```python
from build123d import *

# Parameters (mm, degrees)
BOSS_EXTRUDE1_DEPTH = 18
CIRPATTERN1_COUNT   = 3
SKETCH4_R           = 1.75
CUT_EXTRUDE1_DEPTH  = 12
CIRPATTERN2_COUNT   = 3
SKETCH5_R           = 1.75
CUT_EXTRUDE2_DEPTH  = 44.819230938
CIRPATTERN3_COUNT   = 3


with BuildPart() as part:
    # Sketch2 → Revolve1 (revolve)
    with BuildSketch(Plane(origin=(0, 0, 0), x_dir=(0, 0, -1), z_dir=(1, 0, 0)), mode=Mode.PRIVATE) as revolve1_sk:
        Polygon((0, 28.25), (-3, 28.25), (-3, 18.5), (0, 18.5), (4, 18.5), (4, 28.25), align=None)
    revolve(revolve1_sk.sketch.rotate(Axis((0, 0, 0), (0, 0, 1)), 90), axis=Axis((0, 0, 0), (0, 0, 1)))

    # Sketch3 → Boss-Extrude1 (add)
    with BuildSketch(Plane.XY.offset(3)):
        with BuildLine():
            Line((-7.524627897, 16.900590966), (-11.490310167, 25.807659178))
            ThreePointArc((-11.490310167, 25.807659178), (0, 28.25), (11.490310167, 25.807659178))
            Line((11.490310167, 25.807659178), (7.524627897, 16.900590966))
            ThreePointArc((7.524627897, 16.900590966), (0, 18.5), (-7.524627897, 16.900590966))
        make_face()
    boss_extrude1 = extrude(amount=BOSS_EXTRUDE1_DEPTH)

    # CirPattern1: Boss-Extrude1 ×3 about axis
    cirpattern1_axis = Axis((0, 0, 0), (0, 0, 1))
    for i in range(1, CIRPATTERN1_COUNT):
        add(boss_extrude1.rotate(cirpattern1_axis, i * 360 / CIRPATTERN1_COUNT))

    # Sketch4 → Cut-Extrude1 (cut)
    with BuildSketch(Plane.XY.offset(21)):
        with Locations((0, 23.25)):
            Circle(SKETCH4_R)
    cut_extrude1 = extrude(amount=-CUT_EXTRUDE1_DEPTH, mode=Mode.SUBTRACT)

    # CirPattern2: Cut-Extrude1 ×3 about axis
    cirpattern2_axis = Axis((0, 0, 0), (0, 0, 1))
    for i in range(1, CIRPATTERN2_COUNT):
        add(cut_extrude1.rotate(cirpattern2_axis, i * 360 / CIRPATTERN2_COUNT), mode=Mode.SUBTRACT)

    # Sketch5 → Cut-Extrude2 (cut, through all)
    with BuildSketch(Plane.XY.offset(3)):
        with Locations((0, -23.25)):
            Circle(SKETCH5_R)
    cut_extrude2 = extrude(amount=-CUT_EXTRUDE2_DEPTH, mode=Mode.SUBTRACT)

    # CirPattern3: Cut-Extrude2 ×3 about axis
    cirpattern3_axis = Axis((0, 0, 0), (0, 0, 1))
    for i in range(1, CIRPATTERN3_COUNT):
        add(cut_extrude2.rotate(cirpattern3_axis, i * 360 / CIRPATTERN3_COUNT), mode=Mode.SUBTRACT)


solid = part.part
```
Design review of the part built by this model. Coordinates are the model's own, in mm. A direction names the side the tool comes from. Coordinates: 2 decimals unless noted, no trailing zeros. Order: outer loops, then holes, each group sorted by start corner. A loop starts at its lowest first (then second) coordinate and runs counter-clockwise, first axis right, second up.
1) Take a section at A-A, the plane z = 8. Give the boundary of the cut face in (x, y), and give its area (3 significant figures).
2) Take a section at C-C, the plane x = -3.5. Give the boundary of the cut face in (y, z), and give its area (3 significant figures).
3) Take a section at D-D, the plane z = 14. Give the boundary of the cut face in (x, y) (3 decimals), and give its area (3 significant figures).
4) Clearance check with flat-ended pins moving along their axes: pin 1 (6 mm diameter, centred on y = 15.5, z = 3, fed in from -X); pin 2 (3 mm diameter, centred on x = 20.14, y = 11.62, fed in from +Z) (3 decimals); pin 3 (4 mm diameter, centred on y = -22, z = 3, fed in from -X); pin 4 (2 mm diameter, centred on y = -16, z = 0, fed in from +X). State where each tip first meets the part, or that it passes through.
5) Mouldability with a two-part tool opening along Y and no side actions: class faces 4 (the flat face through (-23.31, -2.45, 11.87)), 5 (the flat face through (0, 23, 9)), 6 (the flat face through (13.78, -18.966, 11.874)), 7 (the flat face through (-22, -12, 21)) as +Y half, -Y half, draft (parallel to the pull), parting line (faces both ways), or undercut.
6) For faces 1 (the cylindrical face through (18.387, -11.548, 15.084)), 2 (the flat face through (23.179, -2.436, 11.874)), 3 (the flat face through (0, -20, 3)), list the 3-axis set-ups (+Z, -Z, +X, -X, +Y, -Y) from which the entire face can be reached by the end or side of a thin tool; tool diameter is ignored.
7) Take a section at B-B, the plane y = 0. Give the boundary of the cut face in (x, z).
8) Wall thickness on line 1 along Y through (x, z) = (0, -2.25); line 2 along Y through (x, z) = (-0.5, -2); line 3 along Z through (x, y) = (-21, -1.5): over which ranges is each line inside the solid? List them lowest first.
Returned:
1. outline: (-28.1, -2.95) arc R28.25 ccw to (-16.6, -22.85) - (-10.87, -14.97) arc R18.5 cw to (-18.4, -1.93) - close; (-11.49, 25.81) - (-7.52, 16.9) arc R18.5 cw to (7.52, 16.9) - (11.49, 25.81) arc R28.25 ccw to start; (10.87, -14.97) - (16.6, -22.85) arc R28.25 ccw to (28.1, -2.95) - (18.4, -1.93) arc R18.5 cw to start
1. area: 573 mm2
2. outline: (-28.03, -4) - (-18.17, -4) - (-18.17, 3) - (-28.03, 3) - close; (18.17, -4) - (28.03, -4) - (28.03, 21) - (18.17, 21) - close
2. area: 316 mm2
3. outline: (-28.095, -2.953) arc R28.25 ccw to (-16.605, -22.855) - (-10.874, -14.967) arc R18.5 cw to (-18.399, -1.934) - close; (-11.49, 25.808) - (-7.525, 16.901) arc R18.5 cw to (7.525, 16.901) - (11.49, 25.808) arc R28.25 ccw to start; (10.874, -14.967) - (16.605, -22.855) arc R28.25 ccw to (28.095, -2.953) - (18.399, -1.934) arc R18.5 cw to start; hole circle Ø3.5 at (-20.135, -11.625); hole circle Ø3.5 at (0, 23.25); hole circle Ø3.5 at (20.135, -11.625)
3. area: 544 mm2
4. pin 1: stops at x = -25.33
4. pin 2: passes through
4. pin 3: stops at x = -19.95
4. pin 4: stops at x = 23.94
5. face 4: +Y half
5. face 5: undercut
5. face 6: -Y half
5. face 7: draft
6. face 1: +Z
6. face 2: +Z, +X, +Y
6. face 3: +Z, -Y
7. outline: (-28.25, -4) - (-18.5, -4) - (-18.5, 3) - (-28.25, 3) - close; (18.5, -4) - (28.25, -4) - (28.25, 3) - (18.5, 3) - close
8. line 1: y = -28.25 to -25, -21.5 to -18.5, 18.5 to 28.25
8. line 2: y = -28.25 to -24.93, -21.57 to -18.49, 18.49 to 28.25
8. line 3: z = -4 to 3
